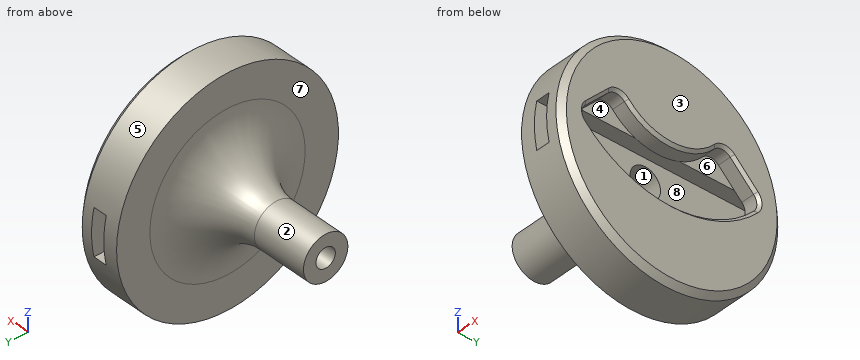
```python
from build123d import *

# Parameters (mm, degrees)
CORTAR_EXTRUIR1_DEPTH = 2.9
REDONDEO1_R           = 10
CORTAR_EXTRUIR2_REACH = 41.799
CROQUIS3_R            = 1.75
CROQUIS4_R            = 2.75
CORTAR_EXTRUIR3_DEPTH = 22.1
CHAFL_N1_SIZE         = 1
CHAFL_N2_SIZE         = 0.5
CROQUIS6_W            = 2.5
CROQUIS6_H            = 8.35
CORTAR_EXTRUIR5_DEPTH = 25


with BuildPart() as part:
    # Croquis1 → Revolución1 (revolve)
    with BuildSketch(Plane.XY):
        Polygon((-20, 0), (-20, 4), (0, 4), (0, 20), (8, 20), (8, 0), align=None)
    revolve(axis=Axis((8, 0, 0), (-1, 0, 0)))

    # Croquis2 → Cortar-Extruir1 (cut)
    with BuildSketch(Plane(origin=(8, 0, 0), x_dir=(0, 0, -1), z_dir=(1, 0, 0))):
        with BuildLine():
            Line((-2.839199656, 15.194118815), (-7.049029232, 10.984289239))
            ThreePointArc((-7.049029232, 10.984289239), (-7.634375098, 9.528098398), (-6.988431485, 8.097756342))
            ThreePointArc((-6.988431485, 8.097756342), (-3.433318471, 0), (-6.988431485, -8.097756342))
            ThreePointArc((-6.988431485, -8.097756342), (-7.634375098, -9.528098398), (-7.049029232, -10.984289239))
            Line((-7.049029232, -10.984289239), (-2.839199656, -15.194118815))
            ThreePointArc((-2.839199656, -15.194118815), (-1.453779812, -15.779697972), (-0.052075025, -15.234248815))
            ThreePointArc((-0.052075025, -15.234248815), (6.516681529, 0), (-0.052075025, 15.234248815))
            ThreePointArc((-0.052075025, 15.234248815), (-1.453779812, 15.779697972), (-2.839199656, 15.194118815))
        make_face()
    extrude(amount=-CORTAR_EXTRUIR1_DEPTH, mode=Mode.SUBTRACT)

    # Redondeo1
    redondeo1_edges = [part.edges().sort_by_distance(p)[0] for p in [
        (0, -4, 0),
    ]]
    fillet(redondeo1_edges, radius=REDONDEO1_R)

    # Croquis3 → Cortar-Extruir2 (cut, up to next)
    with BuildSketch(Plane.ZY.offset(20), mode=Mode.PRIVATE) as cortar_extruir2_sk1:
        with Locations(Location((0, 0, 0), (0, 0, 270))):
            Circle(CROQUIS3_R)
    cortar_extruir2_tool1 = extrude(cortar_extruir2_sk1.sketch, amount=-CORTAR_EXTRUIR2_REACH, mode=Mode.PRIVATE) & part.part
    add(cortar_extruir2_tool1.solids().sort_by_distance((-20, 0, 0))[0], mode=Mode.SUBTRACT)

    # Croquis4 → Cortar-Extruir3 (cut)
    with BuildSketch(Plane(origin=(5.1, 0, 0), x_dir=(0, 0, -1), z_dir=(1, 0, 0))):
        with Locations(Location((0, 0, 0), (0, 0, 90))):
            Circle(CROQUIS4_R)
    extrude(amount=-CORTAR_EXTRUIR3_DEPTH, mode=Mode.SUBTRACT)

    # Chaflán1
    chafl_n1_edges = [part.edges().sort_by_distance(p)[0] for p in [
        (8, -20, 0),
    ]]
    chamfer(chafl_n1_edges, length=CHAFL_N1_SIZE)

    # Chaflán2
    chafl_n2_edges = [part.edges().sort_by_distance(p)[0] for p in [
        (8, -15.779697972, 1.453779812),
        (8, 0, -6.516681529),
        (8, 15.779697972, 1.453779812),
        (8, 13.089204027, 4.944114444),
        (8, 9.528098398, 7.634375098),
        (8, 0, 3.433318471),
        (8, -9.528098398, 7.634375098),
        (8, -13.089204027, 4.944114444),
    ]]
    chamfer(chafl_n2_edges, length=CHAFL_N2_SIZE)

    # Croquis6 → Cortar-Extruir5 (cut, symmetric)
    with BuildSketch(Plane(origin=(0, 0, 0), x_dir=(1, 0, 0), z_dir=(0, 1, 0))):
        with Locations((3.85, 0)):
            Rectangle(CROQUIS6_W, CROQUIS6_H)
    extrude(amount=CORTAR_EXTRUIR5_DEPTH, both=True, mode=Mode.SUBTRACT)


solid = part.part
```
The listing builds one solid part. Answer for the finished solid, in the listing's coordinates (mm). Face numbers are marked on the shaded views. A direction names the side the tool comes from. Round coordinates to 2 decimals unless told otherwise and drop trailing zeros. Order: outer loops, then holes, each group sorted by start corner. A loop starts at its lowest first (then second) coordinate and runs counter-clockwise, first axis right, second up. Notation, with made-up numbers: (1, 75) - (44, 75) arc R29 cw to (44, 102) - close; hole circle Ø6 at (86.25, 47). An arc over 180 degrees is marked (long way). Put each result on its own line as item: value. Start each with the question number.
(1) Determine the mould class of the marked faces 1, 2, 3 and 4 for opening direction Y: released by +Y, released by -Y, zero draft, split by the parting line, or undercut.
(2) Find section C-C (x = -4). Give the vertices of the cut face in (y, z).
(3) Straight lines are drawn through the part: probe 1 along Z at (x, y) = (-18.75, 0); probe 2 along Y at (x, z) = (6, 5); probe 3 along X at (y, z) = (12.5, 12). For each, find the intervals that lie inside material, in ascending order. Write a range as from..to.
(4) Find section A-A (x = -15). Give the vertices of the cut face in (y, z).
(5) For the marked faces 5, 6, 7 and 8, determine the directions among +Z, -Z, +X, -X, +Y, -Y from which every point of the face is accessible in a straight line to the end or side of a thin tool.
(6) Given P1, Ø12, axis at x = 2.5, y = 13, coming from the +Z side (3 decimals); P2, Ø5, axis at x = -7, z = -2, coming from the +Y side; P3, Ø9, axis at y = 10, z = 1, coming from the +X side; P4, Ø2, axis at y = 0, z = 0, coming from the -X side, each flat-ended and moving along its own axis, determine where each tip first touches the part or whether it passes through.
Reply:
1. face 1: undercut
1. face 2: split by the parting line
1. face 3: zero draft
1. face 4: undercut
2. outline: circle Ø12 at (0, 0); hole circle Ø5.5 at (0, 0)
3. probe 1: -4..-1.75, 1.75..4
3. probe 2: -19.36..-13.03, -5.66..5.66, 13.03..19.36
3. probe 3: 0..8
4. outline: circle Ø8 at (0, 0); hole circle Ø5.5 at (0, 0)
5. face 5: +X, -X
5. face 6: +X
5. face 7: -X
5. face 8: +Y, -Y
6. P1: z = 18.735
6. P2: y = 5.43
6. P3: x = 7.8
6. P4: through
